```python
from build123d import *

# Parameters (mm, degrees)
SKETCH1_R                  = 10.5
BOSS_EXTRUDE1_DEPTH        = 18
SKETCH3_R                  = 0.487346303
BOSS_EXTRUDE2_DEPTH        = 0.8
M5_TAPPED_HOLE1_AT_2_COUNT = 2
M5_TAPPED_HOLE1_AT_2_PITCH = 26
M5_TAPPED_HOLE1_AT_3_COUNT = 2
M5_TAPPED_HOLE1_AT_3_PITCH = 30.5
M5_TAPPED_HOLE1_AT_4_COUNT = 2
M5_TAPPED_HOLE1_AT_4_PITCH = 40.078048855
CHAMFER1_SIZE              = 0.2
CHAMFER1_SIZE2             = 0.346410162
CHAMFER1_PART_2_SIZE       = 0.2
CHAMFER1_PART_2_SIZE2      = 0.346410162


with BuildPart() as part:
    # Sketch1 → Boss-Extrude1 (new body, symmetric)
    with BuildSketch(Plane.XY):
        Polygon((-9, -1), (9, -1), (11, 0), (21, 0), (21, -8), (19.5, -12), (19.5, -24), (11, -24), (7.5, -28), (-7.5, -28), (-11, -24), (-19.5, -24), (-19.5, -12), (-21, -8), (-21, 0), (-11, 0), align=None)
        with Locations((0, -15)):
            Circle(SKETCH1_R, mode=Mode.SUBTRACT)
    extrude(amount=BOSS_EXTRUDE1_DEPTH, both=True)

    # Sketch2 → Revolve1 (revolve)
    with BuildSketch(Plane(origin=(0, 0, 0), x_dir=(0, 0, -1), z_dir=(1, 0, 0))):
        Polygon((-15, -4.5), (15, -4.5), (15, -5.6), (14.2, -5.6), (14.2, -8.2), (14.8, -8.2), (14.8, -9), (-14.8, -9), (-14.8, -8.2), (-14.2, -8.2), (-14.2, -5.6), (-15, -5.6), align=None)
    revolve(axis=Axis((0, -15, 30.2753079), (0, 0, -1)))

    # Sketch3 → Boss-Extrude2 (add)
    with BuildSketch(Plane.XY.offset(15)):
        with BuildLine():
            Line((1.141194716, -4.059356755), (0.782998979, -5.534631753))
            ThreePointArc((0.782998979, -5.534631753), (1.493962208, -6.63757679), (2.559436926, -5.871600228))
            ThreePointArc((2.559436926, -5.871600228), (0, -23.5), (-2.559436926, -5.871600228))
            ThreePointArc((-2.559436926, -5.871600228), (-1.493962208, -6.63757679), (-0.782998979, -5.534631753))
            Line((-0.782998979, -5.534631753), (-1.141194716, -4.059356755))
            ThreePointArc((-1.141194716, -4.059356755), (0, -26), (1.141194716, -4.059356755))
        make_face()
        with Locations((1.662663475, -5.748213677)):
            Circle(SKETCH3_R, mode=Mode.SUBTRACT)
        with Locations((-1.662663475, -5.748213677)):
            Circle(SKETCH3_R, mode=Mode.SUBTRACT)
    boss_extrude2 = extrude(amount=BOSS_EXTRUDE2_DEPTH)

    # Mirror1: Boss-Extrude2 across plane
    add(boss_extrude2.mirror(Plane.XY))

    # Sketch6 → M5 Tapped Hole1 (revolve, cut)
    with BuildSketch(Plane(origin=(15.25, 0, -13), x_dir=(0, 0, 1), z_dir=(1, 0, 0))):
        Polygon((0, 0), (0, 24), (2.5, 24), (2.1, 23.6), (2.1, 12), (2.5, 12), (2.5, 0), align=None)
    m5_tapped_hole1 = revolve(axis=Axis((15.25, 6.35, -13), (0, -1, 0)), mode=Mode.SUBTRACT)

    # M5 Tapped Hole1 at 2: M5 Tapped Hole1 ×2
    with Locations(*[(0, 0, i * M5_TAPPED_HOLE1_AT_2_PITCH) for i in range(1, M5_TAPPED_HOLE1_AT_2_COUNT)]):
        add(m5_tapped_hole1, mode=Mode.SUBTRACT)

    # M5 Tapped Hole1 at 3: M5 Tapped Hole1 ×2
    with Locations(*[(-i * M5_TAPPED_HOLE1_AT_3_PITCH, 0, 0) for i in range(1, M5_TAPPED_HOLE1_AT_3_COUNT)]):
        add(m5_tapped_hole1, mode=Mode.SUBTRACT)

    # M5 Tapped Hole1 at 4: M5 Tapped Hole1 ×2
    with Locations(*[Vector(-0.761015091, 0, 0.648734176) * (i * M5_TAPPED_HOLE1_AT_4_PITCH) for i in range(1, M5_TAPPED_HOLE1_AT_4_COUNT)]):
        add(m5_tapped_hole1, mode=Mode.SUBTRACT)

    # Chamfer1
    chamfer1_edges = [part.edges().sort_by_distance(p)[0] for p in [
        (-10.5, -15, -18),
    ]]
    chamfer1_side = [part.faces().sort_by_distance(p)[0] for p in [
        (-10.5, -15, -16.5),
    ]]
    chamfer(chamfer1_edges, length=CHAMFER1_SIZE, length2=CHAMFER1_SIZE2, reference=chamfer1_side[0])

    # Chamfer1 part 2
    chamfer1_part_2_edges = [part.edges().sort_by_distance(p)[0] for p in [
        (-10.5, -15, 18),
    ]]
    chamfer1_part_2_side = [part.faces().sort_by_distance(p)[0] for p in [
        (0, -1.504777179, 18),
    ]]
    chamfer(chamfer1_part_2_edges, length=CHAMFER1_PART_2_SIZE, length2=CHAMFER1_PART_2_SIZE2, reference=chamfer1_part_2_side[0])


solid = part.part
```
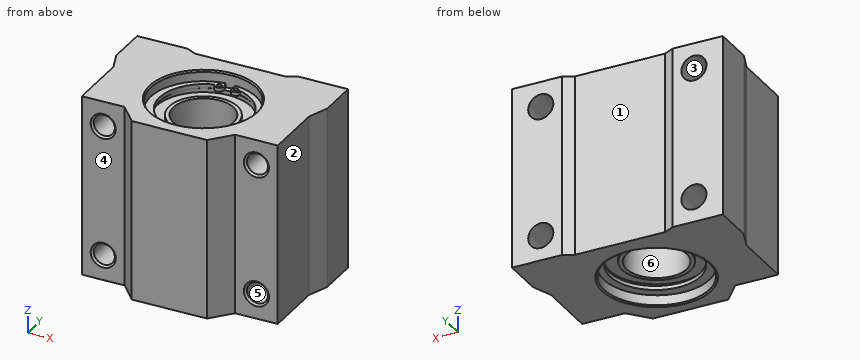
Build history of the part. All positions in model axes, mm. Face numbers are marked on the shaded views. A direction names the side the tool comes from. Coordinates: 2 decimals unless noted, no trailing zeros. Order: outer loops, then holes, each group sorted by start corner. A loop starts at its lowest first (then second) coordinate and runs counter-clockwise, first axis right, second up. Notation, with made-up numbers: (55, 16) -> (105, 16) arc R25 cw to (105, 29) -> close; hole circle Ø6 at (0.25, 17.25). An arc over 180 degrees is marked (long way). Answer in a Markdown table with one row per item. Add a question column.
Q1. Band-saw the part on B-B, the plane z = 10. List the corners of the cut face in (x, y), then the cut area to 3 significant figures.
Q2. Band-saw the part on C-C, the plane y = -15. Give the number of separate pieces and of enclosed holes in the cut face, then the cut area to 3 significant figures.
Q3. Band-saw the part on A-A, the plane x = 15.25. List the corners of the cut face in (y, z), then the cut area to 3 significant figures.
Q4. Mould opens along Y. For the marked faces 4, 5 and 6 say: +Y half, -Y half, draft (parallel to the pull), parting line (faces both ways), or undercut.
Q5. Which spindle directions (+Z, -Z, +X, -X, +Y, -Y) get a long thin tool onto all of the face, cutting with end or side? Do the marked faces 1, 2 and 3. Say none if no direction does.
Q6. Wall check: line 1 along X through (y, z) = (-7.75, -13); line 2 along Z through (x, y) = (15.25, -3.75); line 3 along Z through (x, y) = (-9, -13.75). Give the ranges that are in metal, low to high. Write a range as [from, to].
Q7. Drop flat-ended pins along their axis: pin 1 (2 mm diameter, centred on x = 2, y = -8, fed in from -Z); pin 2 (6.5 mm diameter, centred on x = 15.25, z = 13, fed in from -Y); pin 3 (4 mm diameter, centred on y = -13, z = -1, fed in from -X) (3 decimals). Give the stop position or say it passes through.
Answers follow:
| question | item | result |
|---|---|---|
| 1 | outline | (-21, -8) -> (-19.5, -12) -> (-19.5, -24) -> (-11, -24) -> (-7.5, -28) -> (7.5, -28) -> (11, -24) -> (19.5, -24) -> (19.5, -12) -> (21, -8) -> (21, 0) -> (11, 0) -> (9, -1) -> (-9, -1) -> (-11, 0) -> (-21, 0) -> close; hole circle Ø12 at (0, -15) |
| 1 | area | 907 mm^2 |
| 2 | separate pieces | 2 |
| 2 | enclosed holes | 4 |
| 2 | area | 858 mm^2 |
| 3 | outline | (-24, -18) -> (0, -18) -> (0, -15.5) -> (-12, -15.5) -> (-12, -15.1) -> (-23.6, -15.1) -> (-24, -15.5) -> close; (-24, -10.5) -> (-23.6, -10.9) -> (-12, -10.9) -> (-12, -10.5) -> (0, -10.5) -> (0, 10.5) -> (-12, 10.5) -> (-12, 10.9) -> (-23.6, 10.9) -> (-24, 10.5) -> close; (-24, 15.5) -> (-23.6, 15.1) -> (-12, 15.1) -> (-12, 15.5) -> (0, 15.5) -> (0, 18) -> (-24, 18) -> close |
| 3 | area | 643 mm^2 |
| 4 | face 4 | -Y half |
| 4 | face 5 | draft |
| 4 | face 6 | undercut |
| 5 | face 1 | +Z, -Z, +Y |
| 5 | face 2 | +Z, -Z, +X, -Y |
| 5 | face 3 | +Y |
| 6 | line 1 | [-21, -17.75], [-12.75, 12.75], [17.75, 21] |
| 6 | line 2 | [-18, -15.5], [-10.5, 10.5], [15.5, 18] |
| 6 | line 3 | [-15.8, -15], [-14.2, 14.2], [15, 15.8] |
| 7 | pin 1 | z = -14.8 |
| 7 | pin 2 | y = -24 |
| 7 | pin 3 | x = -19.875 |
